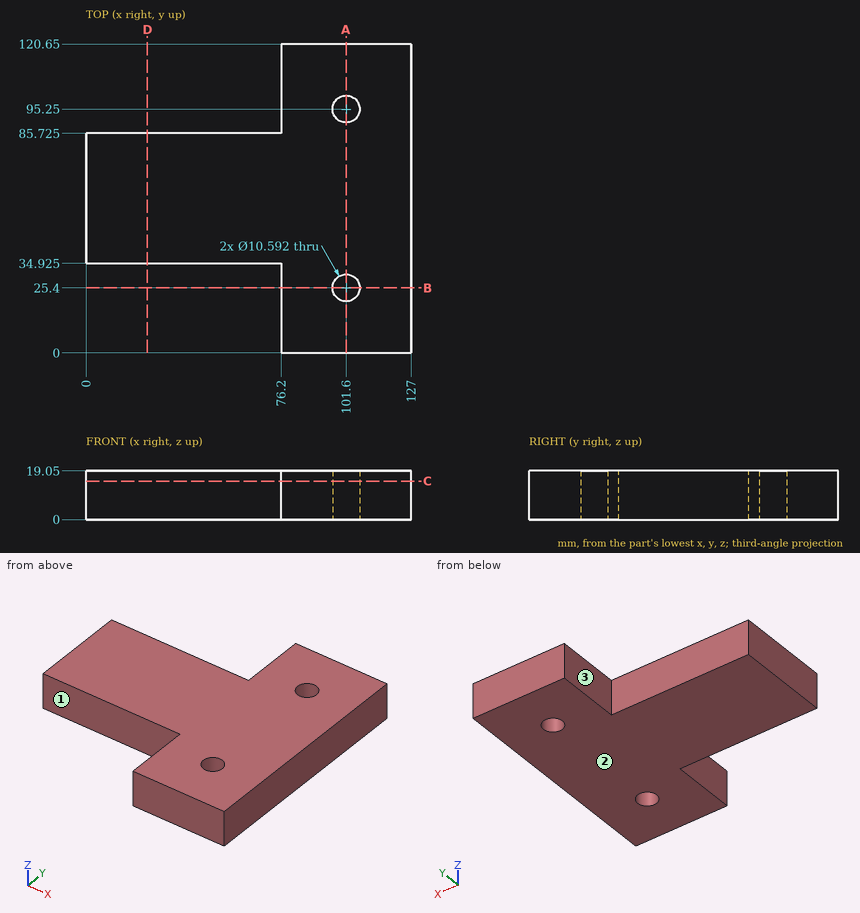
Study the drawing (mm; zero at the part's minimum x, y, z) and answer. A direction names the side the tool comes from. Give positions to 0.01 mm unless a question says otherwise; leave off trailing zeros. Order: outer loops, then holes, each group sorted by start corner. A loop starts at its lowest first (then second) coordinate and runs counter-clockwise, first axis right, second up. Notation, with made-up numbers: (65, 66) -> (116, 66) arc R13 cw to (116, 86) -> close; hole circle Ø10 at (9, 47.25). An arc over 180 degrees is marked (long way). Put each result on its own line as item: value.
Item 1: A cutting plane is placed at A-A on x = 101.6. Give the vertices of the cut face in (y, z), plus the area to 3 significant figures.
Established:
outline: (0, 0) -> (20.1, 0) -> (20.1, 19.05) -> (0, 19.05) -> close; (30.7, 0) -> (89.95, 0) -> (89.95, 19.05) -> (30.7, 19.05) -> close; (100.55, 0) -> (120.65, 0) -> (120.65, 19.05) -> (100.55, 19.05) -> close
area: 1,890 mm^2
Item 2: A cutting plane is placed at B-B on y = 25.4. Give the vertices of the cut face in (x, z), plus the area to 3 significant figures.
Established:
outline: (76.2, 0) -> (96.3, 0) -> (96.3, 19.05) -> (76.2, 19.05) -> close; (106.9, 0) -> (127, 0) -> (127, 19.05) -> (106.9, 19.05) -> close
area: 766 mm^2
Item 3: For the marked faces 1, 2 and 3, determine the directions among +Z, -Z, +X, -X, +Y, -Y from which every point of the face is accessible in a straight line to the end or side of a thin tool.
Established:
face 1: +Z, -Z, -X, -Y
face 2: -Z, +X, -X, +Y, -Y
face 3: +Z, -Z, -X, +Y
Item 4: Given P1, Ø1, axis at y = 78.5, z = 15, coming from the -X side; P2, Ø9.5, axis at y = 21, z = 11.5, coming from the -X side, each flat-ended and moving along its own axis, determine where each tip first touches the part or whether it passes through.
Established:
P1: stops at x = 0
P2: stops at x = 76.2
Item 5: A cutting plane is placed at C-C on z = 15. Count the separate pieces of the cut face and the enclosed holes in it, plus the area to 3 significant figures.
Established:
separate pieces: 1
enclosed holes: 2
area: 9,820 mm^2
Item 6: Straight lines are drawn through the part: line 1 (Y direction, x = 101.6, z = 6.75); line 2 (X direction, y = 25, z = 5.5); line 3 (Y direction, x = 103.5, z = 17.5). For each, find the intervals that lie inside material, in ascending order.
Established:
line 1: y = 0 to 20.1, 30.7 to 89.95, 100.55 to 120.65
line 2: x = 76.2 to 96.32, 106.88 to 127
line 3: y = 0 to 20.46, 30.34 to 90.31, 100.19 to 120.65
Item 7: A cutting plane is placed at D-D on x = 24. Give the vertices of the cut face in (y, z) (3 decimals).
Established:
outline: (34.925, 0) -> (85.725, 0) -> (85.725, 19.05) -> (34.925, 19.05) -> close
